The drawing under review shows one solid part. Ordinate dimensions are in mm from its lowest x, y, z. A direction names the side the tool comes from. Round coordinates to 2 decimals unless told otherwise and drop trailing zeros. Order: outer loops, then holes, each group sorted by start corner. A loop starts at its lowest first (then second) coordinate and runs counter-clockwise, first axis right, second up. Notation, with made-up numbers: (71.5, 84.5) -> (92.5, 84.5) arc R16 cw to (92.5, 105.5) -> close; hole circle Ø1 at (86.5, -38.5). An arc over 180 degrees is marked (long way). Return JSON: item names as keys, results as strings. Group by question number.
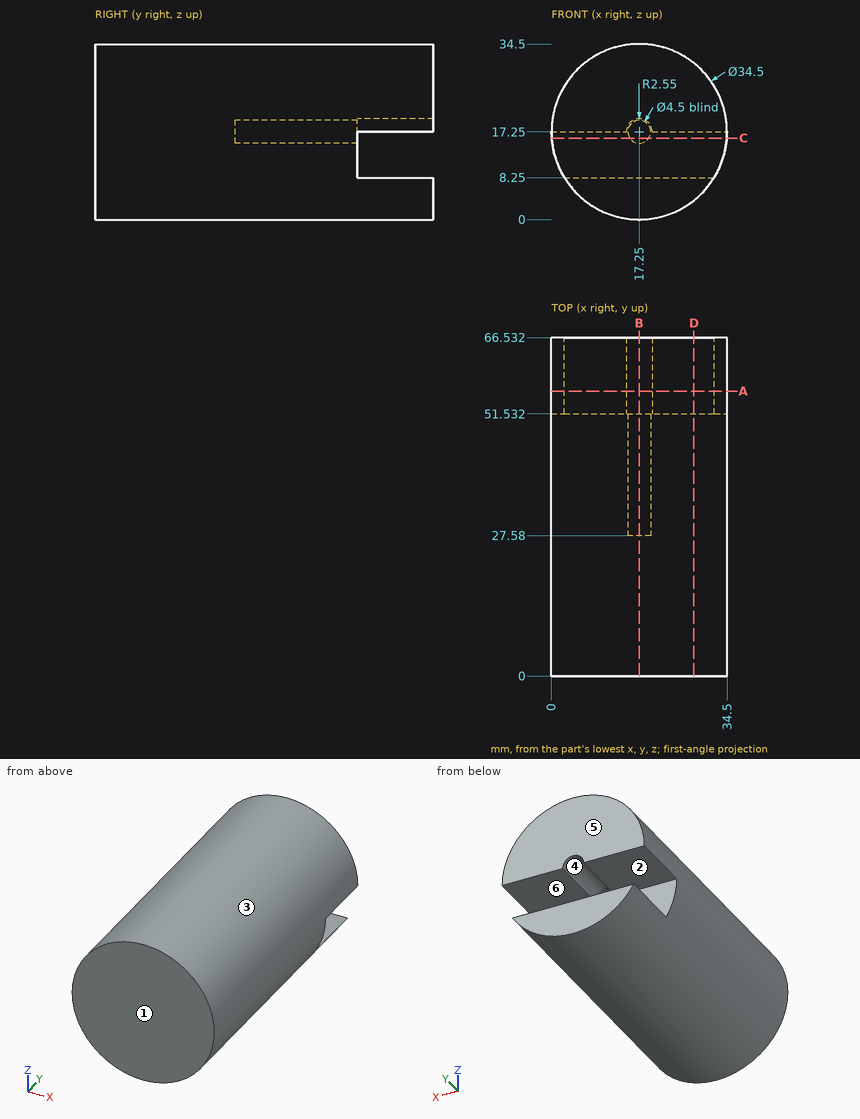
Item 1: Consider section B-B on x = 17.25. State the section outline as (y, z) points, plus the area to 3 significant figures.
Item 2: Consider section D-D on x = 28. State the section outline as (y, z) points.
Item 3: Insertion check: pin 1 Ø3 at (x, y) = (13.5, 10.5) entering from +Z; pin 2 Ø1.5 at (x, y) = (30, 7) entering from -Z; pin 3 Ø3 at (x, z) = (4.5, 14.5) entering from +Y. Each pin has a flat end and moves straight along its axis. Give the tip position at first contact, or say it passes through.
Item 4: Wall thickness on line 1 along X through (y, z) = (45, 17) (1 decimal); line 2 along Y through (x, z) = (18.5, 13.5): over which ranges is each line inside the solid? List them lowest first.
Item 5: The part is to be moulded in two halves that separate along Z. For the marked faces 1, 2 and 3, say which applies: +Z half, -Z half, draft (parallel to the pull), parting line (faces both ways), or undercut.
Item 6: Consider section A-A on y = 56. State the section outline as (x, z) points.
Item 7: Consider section C-C on z = 16. State the section outline as (x, y) points (1 decimal).
Item 8: For the marked faces 4, 5 and 6, list the 3-axis set-ups (+Z, -Z, +X, -X, +Y, -Y) from which the entire face can be reached by the end or side of a thin tool; tool diameter is ignored.
Values:
{
 "1": {"outline": "(0, 0) -> (66.53, 0) -> (66.53, 8.25) -> (51.53, 8.25) -> (51.53, 15) -> (27.58, 15) -> (27.58, 19.5) -> (51.53, 19.5) -> (51.53, 19.8) -> (66.53, 19.8) -> (66.53, 34.5) -> (0, 34.5) -> close", "area": "2,010 mm^2"},
 "2": {"outline": "(0, 3.76) -> (66.53, 3.76) -> (66.53, 8.25) -> (51.53, 8.25) -> (51.53, 17.25) -> (66.53, 17.25) -> (66.53, 30.74) -> (0, 30.74) -> close"},
 "3": {"pin 1": "z = 34.35", "pin 2": "z = 4.86", "pin 3": "y = 51.53"},
 "4": {"line 1": "0 to 15, 19.5 to 34.5", "line 2": "0 to 51.53"},
 "5": {"face 1": "draft", "face 2": "undercut", "face 3": "parting line"},
 "6": {"outline": "(0, 17.25) -> (14.7, 17.25) arc R2.55 cw to (19.8, 17.25) -> (34.5, 17.25) arc R17.25 ccw to start; (2.53, 8.25) arc R17.25 ccw to (31.97, 8.25) -> close"},
 "7": {"outline": "(0, 0) -> (34.5, 0) -> (34.5, 51.5) -> (19.1, 51.5) -> (19.1, 27.6) -> (15.4, 27.6) -> (15.4, 51.5) -> (0, 51.5) -> close"},
 "8": {"face 4": "+Y", "face 5": "+Z, -Z, +X, -X, +Y", "face 6": "+X, -X, +Y"}
}
